Build history of the part. All positions in model axes, mm. Face numbers are marked on the shaded views. Give positions to 0.01 mm unless a question says otherwise; leave off trailing zeros. One line per item, written item: value.
from build123d import *

# Parameters (mm, degrees)
F0_W          = 38.1
F0_H          = 88.9
F1_DEPTH      = 685.8
F1_DEPTH_BACK = 685.8
F2_R          = 3.175
F3_DEPTH      = 12.7
F4_R          = 2.54


# Not quite as in the source:
# - a length typed as a fraction of an inch, garbled in the dataset ("3 / 203.2 mm" for 3/8 in), is restored
# - a pattern or mirror of a feature is missing from the dataset's text; its kind, count and spacing are read off the source's solid


with BuildPart() as f1:
    # F0 (on Front) → F1 (new body, two sides)
    with BuildSketch(Plane.XZ) as f1_sk:
        Rectangle(F0_W, F0_H)
    extrude(amount=F1_DEPTH)
    extrude(f1_sk.sketch, amount=-F1_DEPTH_BACK)

    # F2 (on face) → F3 (cut)
    with BuildSketch(Plane.YZ.offset(19.05)):
        with Locations((-666.75, 22.225)):
            Circle(F2_R)
    f3 = extrude(amount=-F3_DEPTH, mode=Mode.SUBTRACT)

    # F3_copies: F3 across plane
    add(f3.mirror(Plane(origin=(0, 0, 0), x_dir=(0, 0.0333148302, 0.999444907), z_dir=(0, 0.999444907, -0.0333148302))), mode=Mode.SUBTRACT)

    # F3_copies1: F3 across plane
    add(f3.mirror(Plane(origin=(0, 0, 0), x_dir=(-1, 0, 0), z_dir=(0, 0, -1))), mode=Mode.SUBTRACT)

    # F3_copies2: F3 across plane
    add(f3.mirror(Plane.ZX), mode=Mode.SUBTRACT)

    # F4
    f4_edges = [f1.edges().sort_by_distance(p)[0] for p in [
        (19.05, 0, 44.45),
        (-19.05, 0, 44.45),
        (19.05, 0, -44.45),
        (-19.05, 0, -44.45),
    ]]
    fillet(f4_edges, radius=F4_R)


solid = f1.part
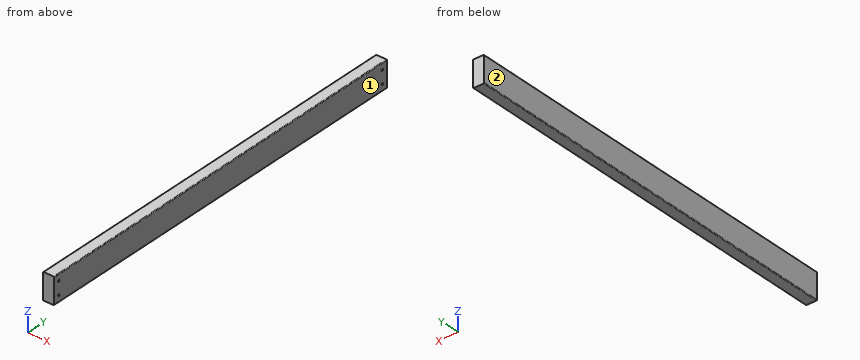
1) Mould opens along X. For the marked faces 1 and 2 say: released by +X, released by -X, zero draft, split by the parting line, or undercut.
Check values:
face 1: released by +X
face 2: released by -X
2) Pin check, flat tip, straight feed: pin 1 (1.9 mm diameter, centred on y = 666.5, z = 23.5, fed in from +X). Stop position of the tip, or through.
Check values:
pin 1: x = 6.35
3) Drill centre lines: probe 1 along Y at (x, z) = (13, 22); probe 2 along Z at (x, y) = (16, -666); probe 3 along Z at (x, y) = (9.75, -666.75). Where is each one in solid material? Low to high. Write a range as from..to.
Check values:
probe 1: -685.8..-669.92, -663.58..663.58, 669.92..685.8
probe 2: -44.45..-25.31, -19.14..19.14, 25.31..44.45
probe 3: -44.45..-25.4, -19.05..19.05, 25.4..44.45
